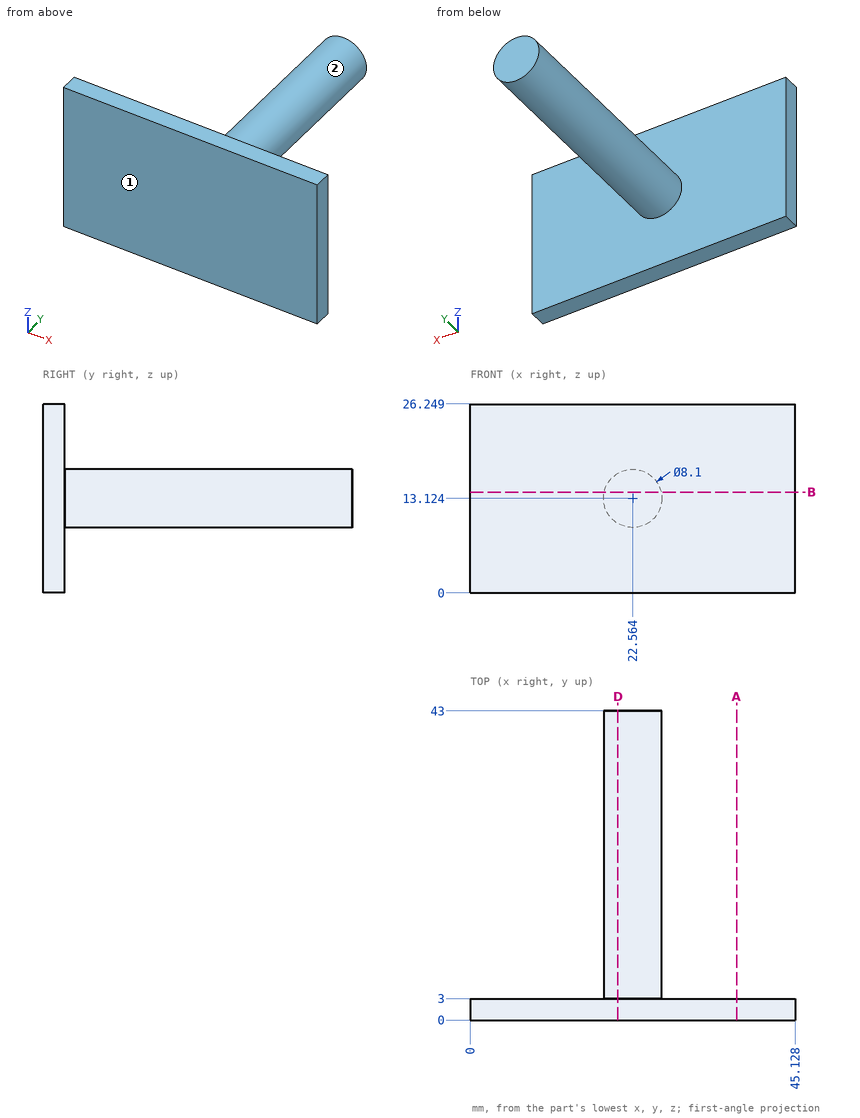
The drawing under review shows one solid part. Ordinate dimensions are in mm from its lowest x, y, z. A direction names the side the tool comes from. Round coordinates to 2 decimals unless told otherwise and drop trailing zeros. Loops run counter-clockwise (first coordinate to the right, second up) from the corner with the lowest first, then second, coordinate; pieces in that order, holes last. Notation, with made-up numbers: (63.25, 38) - (110.25, 38) arc R29 ccw to (110.25, 74) - close; hole circle Ø5 at (31, 24). An arc over 180 degrees is marked (long way). One line per item, written item: value. Start each with the question number.
1) Consider section D-D on x = 20.5. Give the boundary of the cut face in (y, z).
2) Insertion check: pin 1 Ø4 at (y, z) = (21, 13) entering from +X; pin 2 Ø5 at (x, y) = (25.5, 23.5) entering from +Z; pin 3 Ø4 at (x, z) = (16.5, 21) entering from +Y; pin 4 Ø8 at (x, y) = (13.5, 23.5) entering from +Z. Each pin has a flat end and moves straight along its axis. Give the tip position at first contact, or say it passes through.
3) Consider section B-B on z = 14. Give the boundary of the cut face in (x, y), then the cut area to 3 significant figures.
4) Consider section A-A on x = 37. Give the boundary of the cut face in (y, z).
5) For the marked faces 1 and 2, list the 3-axis set-ups (+Z, -Z, +X, -X, +Y, -Y) from which the entire face can be reached by the end or side of a thin tool; tool diameter is ignored.
6) To check wall thickness, follow L1, parallel to Y at x = 2.5, z = 7; L2, parallel to X at y = 37.5, z = 14; L3, parallel to X at y = 9.5, z = 16 (1 decimal). State the ranges of each line that lie inside material, in increasing order. Write a range as from..to.
Reported:
1. outline: (0, 0) - (3, 0) - (3, 9.64) - (43, 9.64) - (43, 16.61) - (3, 16.61) - (3, 26.25) - (0, 26.25) - close
2. pin 1: stops at x = 26.61
2. pin 2: stops at z = 17.15
2. pin 3: stops at y = 3
2. pin 4: passes through
3. outline: (0, 0) - (45.13, 0) - (45.13, 3) - (26.52, 3) - (26.52, 43) - (18.61, 43) - (18.61, 3) - (0, 3) - close
3. area: 452 mm^2
4. outline: (0, 0) - (3, 0) - (3, 26.25) - (0, 26.25) - close
5. face 1: +Z, -Z, +X, -X, -Y
5. face 2: +Y
6. L1: y = 0..3
6. L2: x = 18.61..26.52
6. L3: x = 19.7..25.4
